For this review, take the finished solid that the model builds, in its own axes (mm). A direction names the side the tool comes from. Round coordinates to 2 decimals unless told otherwise and drop trailing zeros. Order: outer loops, then holes, each group sorted by start corner. A loop starts at its lowest first (then second) coordinate and runs counter-clockwise, first axis right, second up. Notation, with made-up numbers: (63.25, -23) - (114.25, -23) arc R20 ccw to (114.25, 0) - close; hole circle Ø10 at (-24.75, 55). An arc over 180 degrees is marked (long way). One line per question, with ' | ' between items.
```python
from build123d import *

# Parameters (mm, degrees)
BOSS_EXTRUDE1_DEPTH = 9
SKETCH3_R           = 34
CUT_EXTRUDE1_DEPTH  = 10
SKETCH4_R           = 1.908180832
SKETCH4_R_2         = 1.75
CUT_EXTRUDE2_DEPTH  = 276.178116638


with BuildPart() as part:
    # Sketch2 → Boss-Extrude1 (new body)
    with BuildSketch(Plane.XY):
        Polygon((110.844662491, -190), (110.844662491, -199), (50.844662491, -199), (50.844662491, -190), (-9.155337509, -190), (-9.155337509, -199), (-69.155337509, -199), (-69.155337509, -190), (-139.155337509, -190), (-139.155337509, -120), (-148.155337509, -120), (-148.155337509, -60), (-139.155337509, -60), (-139.155337509, 0), (-148.155337509, 0), (-148.155337509, 60), (-139.155337509, 60), (-139.155337509, 130), (-69.155337509, 130), (-69.155337509, 139), (-9.155337509, 139), (-9.155337509, 130), (50.844662491, 130), (50.844662491, 139), (110.844662491, 139), (110.844662491, 130), (180.844662491, 130), (180.844662491, 60), (189.844662491, 60), (189.844662491, 0), (180.844662491, 0), (180.844662491, -60), (189.844662491, -60), (189.844662491, -120), (180.844662491, -120), (180.844662491, -190), align=None)
    extrude(amount=BOSS_EXTRUDE1_DEPTH)

    # Sketch3 → Cut-Extrude1 (cut)
    with BuildSketch(Plane.XY.offset(9)):
        with Locations((20.844662491, -27.75)):
            Circle(SKETCH3_R)
    extrude(amount=-CUT_EXTRUDE1_DEPTH, mode=Mode.SUBTRACT)

    # Sketch4 → Cut-Extrude2 (cut, through all)
    with BuildSketch(Plane.XY.offset(9)):
        with Locations((69.247698425, -26.871593426)):
            Circle(SKETCH4_R)
        with Locations((-25.819672208, -29.158773424)):
            Circle(SKETCH4_R_2)
    extrude(amount=-CUT_EXTRUDE2_DEPTH, mode=Mode.SUBTRACT)


solid = part.part
```
(1) Insertion check: pin 1 (2.5 mm diameter, centred on x = -99, z = 4.5, fed in from -Y); pin 2 (4.5 mm diameter, centred on y = -192.5, z = 5.5, fed in from +X); pin 3 (3 mm diameter, centred on x = 69.25, y = -26.87, fed in from +Z); pin 4 (4.5 mm diameter, centred on x = -145, z = 5, fed in from -Y). Each pin has a flat end and moves straight along its axis. Give the tip position at first contact, or say it passes through.
Output values:
pin 1: y = -190 | pin 2: x = 110.84 | pin 3: through | pin 4: y = -120
(2) We need section C-C on z = 7.5. Give the number of separate pieces and of enclosed holes in the cut face, plus the area to 3 significant figures.
Output values:
separate pieces: 1 | enclosed holes: 3 | area: 103,000 mm^2
(3) We need section B-B on y = 70.5. State the section outline as (x, z) points.
Output values:
outline: (-139.16, 0) - (180.84, 0) - (180.84, 9) - (-139.16, 9) - close
(4) For probe 1 along Y at (x, z) = (7, 1.25); probe 2 along X at (y, z) = (-5.5, 1.25); probe 3 along Y at (x, z) = (116, 5), list the stretches that pass through material, from the lowest coordinate up. Write a range as [from, to].
Output values:
probe 1: [-190, -58.8], [3.3, 130] | probe 2: [-139.16, -4.86], [46.55, 180.84] | probe 3: [-190, 130]
(5) We need section A-A on x = -80. State the section outline as (y, z) points.
Output values:
outline: (-190, 0) - (130, 0) - (130, 9) - (-190, 9) - close
(6) Mouldability with a two-part tool opening along Y and no side actions: class faces 6 (the flat face through (-9.155, 135, 4)), 7 (the flat face through (-40, 139, 4)), 8 (the flat face through (185, -60, 4)) as released by +Y, released by -Y, zero draft, split by the parting line, or undercut.
Output values:
face 6: zero draft | face 7: released by +Y | face 8: undercut
(7) For faces 1 (the flat face through (50.845, -195, 4)), 2 (the flat face through (185, 0, 4)), 3 (the flat face through (-139.155, -30, 4)), 4 (the flat face through (180.845, -155, 4)), 5 (the flat face through (50.845, 134, 4)), list the 3-axis set-ups (+Z, -Z, +X, -X, +Y, -Y) from which the entire face can be reached by the end or side of a thin tool; tool diameter is ignored.
Output values:
face 1: +Z, -Z, -Y | face 2: +Z, -Z, +X | face 3: +Z, -Z, -X | face 4: +Z, -Z, +X, -Y | face 5: +Z, -Z, +Y
